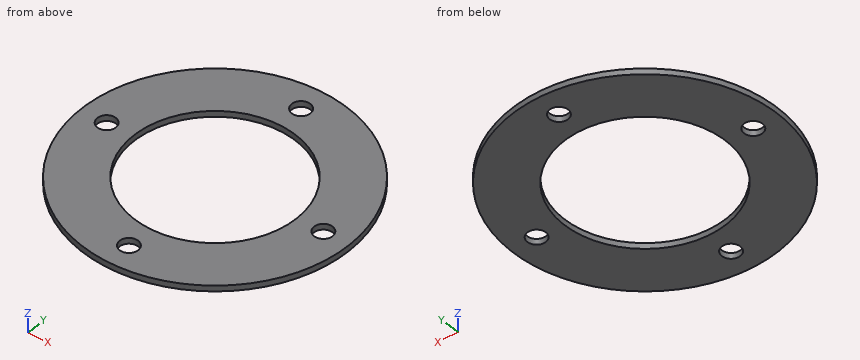
from build123d import *

# Parameters (mm, degrees)
F0_R            = 115
F0_R_2          = 70
F1_DEPTH        = 5
F2_R            = 8
F3_DEPTH        = 25
F3_COPIES_COUNT = 4


# Not quite as in the source:
# - a pattern or mirror of a feature is missing from the dataset's text; its kind, count and spacing are read off the source's solid


with BuildPart() as f1:
    # F0 (on Top) → F1 (new body)
    with BuildSketch(Plane.XY):
        Circle(F0_R)
        Circle(F0_R_2, mode=Mode.SUBTRACT)
    extrude(amount=F1_DEPTH)

    # F2 (on face) → F3 (cut)
    with BuildSketch(Plane.XY.offset(5)):
        with Locations((0, 92.5)):
            Circle(F2_R)
    f3 = extrude(amount=-F3_DEPTH, mode=Mode.SUBTRACT)

    # F3_copies: F3 ×4 about axis
    f3_copies_axis = Axis((0, 0, 0), (0, 0, 1))
    for i in range(1, F3_COPIES_COUNT):
        add(f3.rotate(f3_copies_axis, i * 360 / F3_COPIES_COUNT), mode=Mode.SUBTRACT)


solid = f1.part
The model under review builds one solid part; all positions refer to its coordinate system, in mm. Round coordinates to 2 decimals unless told otherwise and drop trailing zeros. Loops run counter-clockwise (first coordinate to the right, second up) from the corner with the lowest first, then second, coordinate; pieces in that order, holes last. Notation, with made-up numbers: (-33.5, 48) -> (-6.5, 48) arc R14 ccw to (-6.5, 65) -> close; hole circle Ø5 at (6, 85). An arc over 180 degrees is marked (long way). Answer as CSV lines item,"result".
1) Add section D-D on z = 0.9. Write out the cut boundary in (x, y).
Geometry results:
outline,"circle Ø230 at (0, 0); hole circle Ø16 at (-92.5, 0); hole circle Ø140 at (0, 0); hole circle Ø16 at (0, -92.5); hole circle Ø16 at (0, 92.5); hole circle Ø16 at (92.5, 0)"
2) For P1, Ø1, axis at x = 32, z = 2.5, coming from the +Y side, flat-tipped, find the tip position at first contact; note if it passes through.
Geometry results:
P1,"stops at y = 110.6"
3) Add section B-B on y = 18. Write out the cut boundary in (x, z).
Geometry results:
outline,"(-113.58, 0) -> (-67.65, 0) -> (-67.65, 5) -> (-113.58, 5) -> close; (67.65, 0) -> (113.58, 0) -> (113.58, 5) -> (67.65, 5) -> close"
4) Add section C-C on x = 54. Write out the cut boundary in (y, z).
Geometry results:
outline,"(-101.53, 0) -> (-44.54, 0) -> (-44.54, 5) -> (-101.53, 5) -> close; (44.54, 0) -> (101.53, 0) -> (101.53, 5) -> (44.54, 5) -> close"
5) To check wall thickness, follow line 1 along Y through (x, z) = (-2, 1.15); line 2 along Y through (x, z) = (47, 3.95); line 3 along X through (y, z) = (6.5, 3.1). State the ranges of each line that lie inside material, in increasing order. Write a range as from..to.
Geometry results:
line 1,"y = -114.98..-100.25, -84.75..-69.97, 69.97..84.75, 100.25..114.98"
line 2,"y = -104.96..-51.87, 51.87..104.96"
line 3,"x = -114.82..-97.16, -87.84..-69.7, 69.7..87.84, 97.16..114.82"
6) Add section A-A on x = 0. Write out the cut boundary in (y, z), plus the area to 3 significant figures.
Geometry results:
outline,"(-115, 0) -> (-100.5, 0) -> (-100.5, 5) -> (-115, 5) -> close; (-84.5, 0) -> (-70, 0) -> (-70, 5) -> (-84.5, 5) -> close; (70, 0) -> (84.5, 0) -> (84.5, 5) -> (70, 5) -> close; (100.5, 0) -> (115, 0) -> (115, 5) -> (100.5, 5) -> close"
area,"290 mm²"
